Can you work these out from the model? Positions are in its coordinate system, mm. A direction names the side the tool comes from. Round coordinates to 2 decimals unless told otherwise and drop trailing zeros. Order: outer loops, then holes, each group sorted by start corner. A loop starts at its lowest first (then second) coordinate and runs counter-clockwise, first axis right, second up. Notation, with made-up numbers: (67.5, 66.25) -> (104.5, 66.25) arc R21 ccw to (104.5, 101.25) -> close; hole circle Ø6 at (46.25, -20). An arc over 180 degrees is marked (long way). Use a Markdown table: item, result. Add a question column.
Q1. For faces 1 (the face through (-80, 31, 12)), 2 (the face through (21.5, 37, 37)), 3 (the face through (-86, 32, 30)), 4 (the face through (58, 41, 37)), which set-ups out of +Z, -Z, +X, -X, +Y, -Y let a thin tool reach every point of the face, with its end or its side?
Q2. I need wall thicknesses on line 1 along Y through (x, z) = (-78, 12.6); line 2 along Y through (x, z) = (82, 30); line 3 along Y through (x, z) = (14, 22). Which ranges of each line are inside material? Lowest first, please. Write a range as [from, to].
Q3. If we section it at C-C on y = 35.25: List the corners of the cut face in (x, z) for me.
Q4. I'm going to push flat-ended pins straight in: pin 1 Ø12 at (y, z) = (37.5, 30.5) entering from -X; pin 2 Ø1.6 at (x, y) = (11.5, 29.5) entering from +Z; pin 3 Ø1.6 at (y, z) = (30.5, 29.5) entering from -X; pin 4 Ø3 at (x, y) = (12, 44.5) entering from -Z. Where does each tip first touch, or does it pass through?
Q5. If we section it at B-B on z = 25: List the corners of the cut face in (x, y) for me.
Q6. If we section it at D-D on x = -61.5: List the corners of the cut face in (y, z) for me, plus the area to 3 significant figures.
Q7. If we section it at A-A on x = 12: List the corners of the cut face in (y, z) for me, plus the area to 3 significant figures.
Q8. We'd pull the mould along Y, two halves only. Please class faces 5 (the face through (-80, 43, 12)), 6 (the face through (-1, 26, 24)), 7 (the face through (28.5, 37, 37)), 8 (the face through (88.5, 44, 37)): +Y half, -Y half, draft (parallel to the pull), parting line (faces both ways), or undercut.
```python
from build123d import *

# Parameters (mm, degrees)
CYLINDER151_R             = 2.6
CYLINDER151_DEPTH         = 2
CYLINDER146_R             = 2.5
CYLINDER146_DEPTH         = 5
FUSION068_PLACEMENT_ANGLE = 90
CYLINDER143_R             = 2.6
CYLINDER143_DEPTH         = 2
CYLINDER142_R             = 2.5
CYLINDER142_DEPTH         = 5
FUSION067_PLACEMENT_ANGLE = 270
CYLINDER141_R             = 2.6
CYLINDER141_DEPTH         = 2
CYLINDER140_R             = 2.5
CYLINDER140_DEPTH         = 5
FUSION065_PLACEMENT_ANGLE = 90
CYLINDER133_R             = 2.6
CYLINDER133_DEPTH         = 2
CYLINDER132_R             = 2.5
CYLINDER132_DEPTH         = 5
CYLINDER135_R             = 2.6
CYLINDER135_DEPTH         = 2
CYLINDER136_R             = 2.5
CYLINDER136_DEPTH         = 5
CYLINDER131_R             = 2.6
CYLINDER131_DEPTH         = 2
CYLINDER130_R             = 2.5
CYLINDER130_DEPTH         = 5
CYLINDER134_R             = 2.6
CYLINDER134_DEPTH         = 2
CYLINDER137_R             = 2.5
CYLINDER137_DEPTH         = 5
CYLINDER150_R             = 2.6
CYLINDER150_DEPTH         = 2
CYLINDER149_R             = 2.5
CYLINDER149_DEPTH         = 5
FUSION069_PLACEMENT_ANGLE = 90
BOX030_W                  = 177
BOX030_H                  = 7
BOX030_DEPTH              = 29
BOX036_W                  = 7
BOX036_H                  = 15
BOX036_DEPTH              = 55
BOX031_W                  = 177
BOX031_H                  = 7
BOX031_DEPTH              = 55


with BuildPart() as cilindro151:
    # Cylinder151 → Cylinder151 (new body)
    with BuildSketch(Plane.XY.offset(5)):
        Circle(CYLINDER151_R)
    extrude(amount=CYLINDER151_DEPTH)


with BuildPart() as obj1:
    # Cylinder146 → Cylinder146 (new body)
    with BuildSketch(Plane.XY):
        Circle(CYLINDER146_R)
    extrude(amount=CYLINDER146_DEPTH)

    # Fusion068: union Cilindro151
    add(cilindro151.part)


with BuildPart() as obj1_1:
    # Fusion068 placement: moved
    add(obj1.part.moved(Location((88.5, 44.5, 30))).rotate(Axis((88.5, 44.5, 30), (0, -1, 0)), FUSION068_PLACEMENT_ANGLE))


with BuildPart() as cilindro143:
    # Cylinder143 → Cylinder143 (new body)
    with BuildSketch(Plane.XY.offset(5)):
        Circle(CYLINDER143_R)
    extrude(amount=CYLINDER143_DEPTH)


with BuildPart() as obj2:
    # Cylinder142 → Cylinder142 (new body)
    with BuildSketch(Plane.XY):
        Circle(CYLINDER142_R)
    extrude(amount=CYLINDER142_DEPTH)

    # Fusion067: union Cilindro143
    add(cilindro143.part)


with BuildPart() as obj2_1:
    # Fusion067 placement: moved
    add(obj2.part.moved(Location((88.5, 29.5, 30))).rotate(Axis((88.5, 29.5, 30), (0, 1, 0)), FUSION067_PLACEMENT_ANGLE))


with BuildPart() as cilindro141:
    # Cylinder141 → Cylinder141 (new body)
    with BuildSketch(Plane.XY.offset(5)):
        Circle(CYLINDER141_R)
    extrude(amount=CYLINDER141_DEPTH)


with BuildPart() as obj3:
    # Cylinder140 → Cylinder140 (new body)
    with BuildSketch(Plane.XY):
        Circle(CYLINDER140_R)
    extrude(amount=CYLINDER140_DEPTH)

    # Fusion065: union Cilindro141
    add(cilindro141.part)


with BuildPart() as obj3_1:
    # Fusion065 placement: moved
    add(obj3.part.moved(Location((-88.5, 29.5, 30))).rotate(Axis((-88.5, 29.5, 30), (0, 1, 0)), FUSION065_PLACEMENT_ANGLE))


with BuildPart() as cilindro133:
    # Cylinder133 → Cylinder133 (new body)
    with BuildSketch(Plane.XY.offset(5)):
        Circle(CYLINDER133_R)
    extrude(amount=CYLINDER133_DEPTH)


with BuildPart() as obj4:
    # Cylinder132 → Cylinder132 (new body)
    with BuildSketch(Plane.XY):
        Circle(CYLINDER132_R)
    extrude(amount=CYLINDER132_DEPTH)

    # Fusion063: union Cilindro133
    add(cilindro133.part)


with BuildPart() as obj4_1:
    # Fusion063 placement: moved
    add(obj4.part.moved(Location((-78, 29.5, 10))))


with BuildPart() as cilindro135:
    # Cylinder135 → Cylinder135 (new body)
    with BuildSketch(Plane.XY.offset(5)):
        Circle(CYLINDER135_R)
    extrude(amount=CYLINDER135_DEPTH)


with BuildPart() as obj5:
    # Cylinder136 → Cylinder136 (new body)
    with BuildSketch(Plane.XY):
        Circle(CYLINDER136_R)
    extrude(amount=CYLINDER136_DEPTH)

    # Fusion062: union Cilindro135
    add(cilindro135.part)


with BuildPart() as obj5_1:
    # Fusion062 placement: moved
    add(obj5.part.moved(Location((12, 44.5, 10))))


with BuildPart() as cilindro131:
    # Cylinder131 → Cylinder131 (new body)
    with BuildSketch(Plane.XY.offset(5)):
        Circle(CYLINDER131_R)
    extrude(amount=CYLINDER131_DEPTH)


with BuildPart() as obj6:
    # Cylinder130 → Cylinder130 (new body)
    with BuildSketch(Plane.XY):
        Circle(CYLINDER130_R)
    extrude(amount=CYLINDER130_DEPTH)

    # Fusion060: union Cilindro131
    add(cilindro131.part)


with BuildPart() as obj6_1:
    # Fusion060 placement: moved
    add(obj6.part.moved(Location((12, 29.5, 10))))


with BuildPart() as cilindro134:
    # Cylinder134 → Cylinder134 (new body)
    with BuildSketch(Plane.XY.offset(5)):
        Circle(CYLINDER134_R)
    extrude(amount=CYLINDER134_DEPTH)


with BuildPart() as obj7:
    # Cylinder137 → Cylinder137 (new body)
    with BuildSketch(Plane.XY):
        Circle(CYLINDER137_R)
    extrude(amount=CYLINDER137_DEPTH)

    # Fusion061: union Cilindro134
    add(cilindro134.part)


with BuildPart() as obj7_1:
    # Fusion061 placement: moved
    add(obj7.part.moved(Location((-78, 44.5, 10))))


with BuildPart() as cilindro150:
    # Cylinder150 → Cylinder150 (new body)
    with BuildSketch(Plane.XY.offset(5)):
        Circle(CYLINDER150_R)
    extrude(amount=CYLINDER150_DEPTH)


with BuildPart() as fusion073:
    # Cylinder149 → Cylinder149 (new body)
    with BuildSketch(Plane.XY):
        Circle(CYLINDER149_R)
    extrude(amount=CYLINDER149_DEPTH)

    # Fusion069: union Cilindro150
    add(cilindro150.part)


with BuildPart() as fusion073_1:
    # Fusion069 placement: moved
    add(fusion073.part.moved(Location((-88.5, 44.5, 30))).rotate(Axis((-88.5, 44.5, 30), (0, 1, 0)), FUSION069_PLACEMENT_ANGLE))

    # Fusion073: union obj1, obj2, obj3, obj4, obj5, obj6, obj7
    add(obj1_1.part)
    add(obj2_1.part)
    add(obj3_1.part)
    add(obj4_1.part)
    add(obj5_1.part)
    add(obj6_1.part)
    add(obj7_1.part)


with BuildPart() as cubo027:
    # Box030 → Box030 (new body)
    with BuildSketch(Plane(origin=(-88.5, 26, 10), x_dir=(1, 0, 0), z_dir=(0, 0, 1))):
        with Locations((88.5, 3.5)):
            Rectangle(BOX030_W, BOX030_H)
    extrude(amount=BOX030_DEPTH)


with BuildPart() as cubo033:
    # Box036 → Box036 (new body)
    with BuildSketch(Plane(origin=(21.5, 33, 10), x_dir=(1, 0, 0), z_dir=(0, 0, 1))):
        with Locations((3.5, 7.5)):
            Rectangle(BOX036_W, BOX036_H)
    extrude(amount=BOX036_DEPTH)


with BuildPart() as obj8:
    # Box031 → Box031 (new body)
    with BuildSketch(Plane(origin=(-88.5, 41, 10), x_dir=(1, 0, 0), z_dir=(0, 0, 1))):
        with Locations((88.5, 3.5)):
            Rectangle(BOX031_W, BOX031_H)
    extrude(amount=BOX031_DEPTH)

    # Fusion072: union Cubo027, Cubo033
    add(cubo027.part)
    add(cubo033.part)

    # Cut057: cut Fusion073
    add(fusion073_1.part, mode=Mode.SUBTRACT)


solid = obj8.part
```
Answer below:
| question | item | result |
|---|---|---|
| 1 | face 1 | -Z |
| 1 | face 2 | +Z, -Z, -X |
| 1 | face 3 | -X |
| 1 | face 4 | +Z, -Z, +X |
| 2 | line 1 | [26, 27], [32, 33], [41, 42], [47, 48] |
| 2 | line 2 | [26, 26.9], [32.1, 33], [41, 41.9], [47.1, 48] |
| 2 | line 3 | [26, 33], [41, 48] |
| 3 | outline | (21.5, 10) -> (28.5, 10) -> (28.5, 65) -> (21.5, 65) -> close |
| 4 | pin 1 | x = -88.5 |
| 4 | pin 2 | z = 39 |
| 4 | pin 3 | x = -81.5 |
| 4 | pin 4 | z = 17 |
| 5 | outline | (-88.5, 26) -> (88.5, 26) -> (88.5, 33) -> (28.5, 33) -> (28.5, 41) -> (88.5, 41) -> (88.5, 48) -> (-88.5, 48) -> (-88.5, 41) -> (21.5, 41) -> (21.5, 33) -> (-88.5, 33) -> close |
| 6 | outline | (26, 10) -> (33, 10) -> (33, 39) -> (26, 39) -> close; (41, 10) -> (48, 10) -> (48, 65) -> (41, 65) -> close |
| 6 | area | 588 mm² |
| 7 | outline | (26, 10) -> (27, 10) -> (27, 15) -> (26.9, 15) -> (26.9, 17) -> (32.1, 17) -> (32.1, 15) -> (32, 15) -> (32, 10) -> (33, 10) -> (33, 39) -> (26, 39) -> close; (41, 10) -> (42, 10) -> (42, 15) -> (41.9, 15) -> (41.9, 17) -> (47.1, 17) -> (47.1, 15) -> (47, 15) -> (47, 10) -> (48, 10) -> (48, 65) -> (41, 65) -> close |
| 7 | area | 517 mm² |
| 8 | face 5 | undercut |
| 8 | face 6 | -Y half |
| 8 | face 7 | undercut |
| 8 | face 8 | draft |
